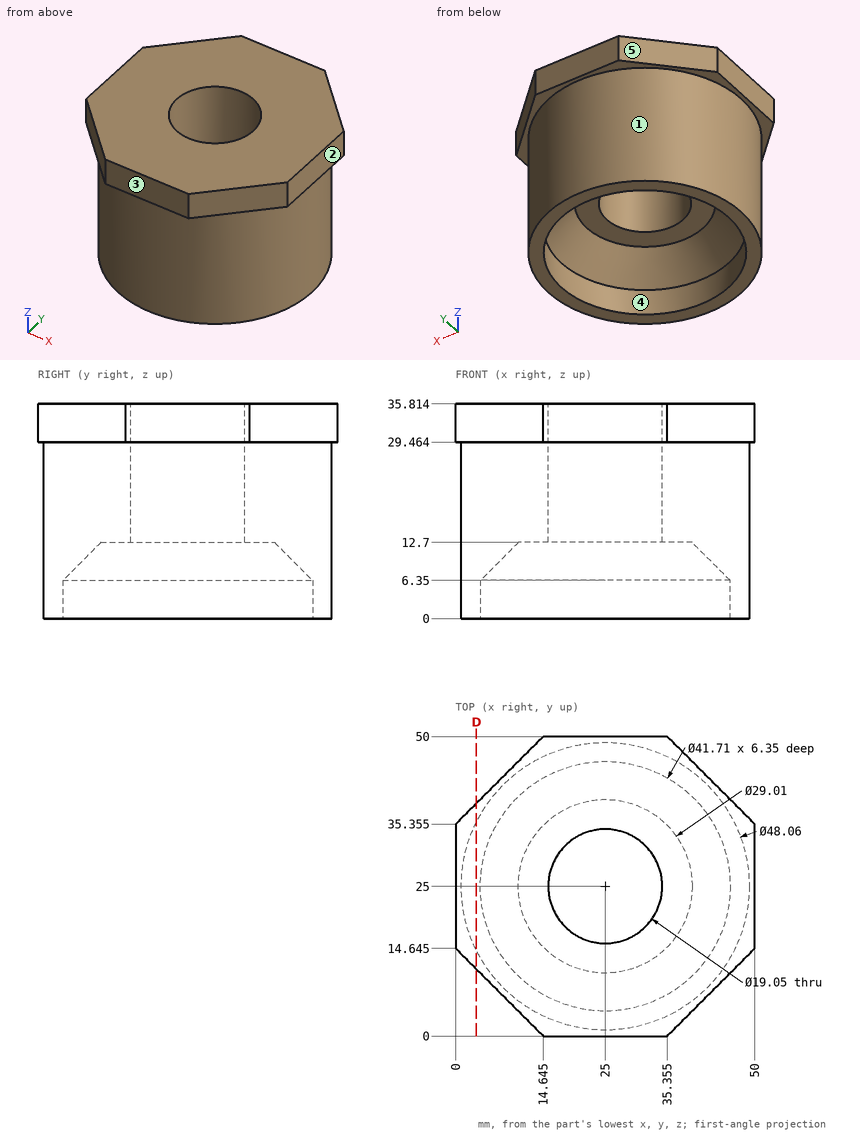
Verification items for this drawing (mm, ordinates from the low corner). A direction names the side the tool comes from. Give positions to 0.01 mm unless a question says otherwise; leave off trailing zeros. Write each loop counter-clockwise with the first axis right and the second up, starting at its lowest first coordinate (ties: lowest second). Pieces come first, ordered by that corner, then holes.
1) Release check for a two-part mould opening along X. For the marked faces 3, 4 and 5 record: released by +X, released by -X, zero draft, split by the parting line, or undercut.
Values follow:
face 3: zero draft
face 4: undercut
face 5: released by -X
2) Cross-section at D-D (x = 3.5). Record the boundary of the cut face in (y, z) (1 decimal).
Values follow:
outline: (11.1, 29.5) - (14.3, 29.5) - (14.3, 0) - (35.7, 0) - (35.7, 29.5) - (38.9, 29.5) - (38.9, 35.8) - (11.1, 35.8) - close
3) Go/stop test with flat-tipped pins: pin 1 Ø4 at (x, y) = (32, 22) entering from -Z; pin 2 Ø1 at (x, z) = (13, 20.5) entering from -Y; pin 3 Ø10 at (y, z) = (35, 20.5) entering from -X; pin 4 Ø12 at (x, y) = (12, 11.5) entering from -Z. Record where each tip stops, or that it passes through.
Values follow:
pin 1: stops at z = 12.7
pin 2: stops at y = 3.9
pin 3: stops at x = 1.5
pin 4: stops at z = 0
4) Thickness scan on line 1 (Y direction, x = 25, z = 29) (1 decimal); line 2 (X direction, y = 25, z = 5) (1 decimal). Record the ranges inside material, lowest first.
Values follow:
line 1: y = 1 to 15.5, 34.5 to 49
line 2: x = 1 to 4.1, 45.9 to 49
5) Set-up check for the marked faces 1 and 2: record each of +Z, -Z, +X, -X, +Y, -Y from which the full face is reachable in a straight line by a thin tool's end or side.
Values follow:
face 1: -Z
face 2: +Z, -Z, +X, +Y, -Y
